For this review, take the finished solid that the model builds, in its own axes (mm). Give positions to 0.01 mm unless a question says otherwise; leave off trailing zeros. Order: outer loops, then holes, each group sorted by start corner. A loop starts at its lowest first (then second) coordinate and runs counter-clockwise, first axis right, second up. Notation, with made-up numbers: (82, 84.5) - (105, 84.5) arc R5 ccw to (105, 90.5) - close; hole circle Ø2 at (-20.75, -32.5). An arc over 180 degrees is marked (long way). Put each result on its own line as item: value. Start each with the question number.
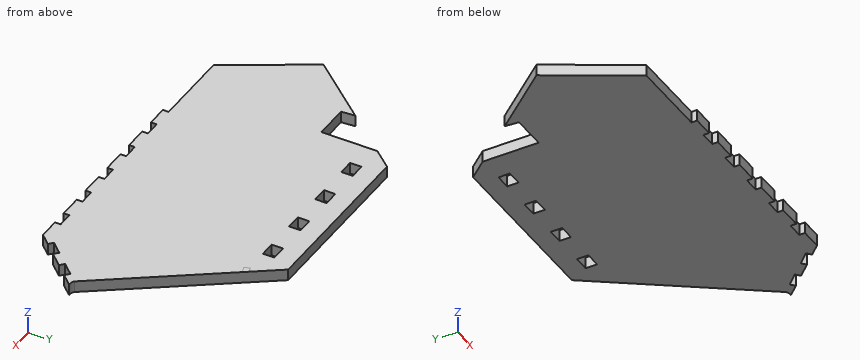
```python
from build123d import *

# Parameters (mm, degrees)
BOSS_EXTRU_1_DEPTH      = 6
ESQUISSE3_W             = 8
ESQUISSE3_H             = 3
ENL_V_MAT_EXTRU_1_DEPTH = 6
BOSS_EXTRU_2_DEPTH      = 6
ENL_V_MAT_EXTRU_2_DEPTH = 6
ENL_V_MAT_EXTRU_3_DEPTH = 10
ESQUISSE9_W             = 8
ESQUISSE9_H             = 6
ENL_V_MAT_EXTRU_4_DEPTH = 6
ENL_V_MAT_EXTRU_5_DEPTH = 10
ENL_V_MAT_EXTRU_6_DEPTH = 0.006


with BuildPart() as part:
    # Esquisse1 → Boss.-Extru.1 (new body)
    with BuildSketch(Plane.XY):
        Polygon((0, 0), (110, 0), (137.279934402, 29.254148065), (105.119046883, 134.447671221), (102.250132615, 133.570556107), (133.904617487, 30.033401375), (108.695562875, 3), (0, 3), align=None)
    extrude(amount=BOSS_EXTRU_1_DEPTH)

    # Esquisse3 → Enl_v. mat.-Extru.1 (cut)
    with BuildSketch(Plane(origin=(0, 0, 0), x_dir=(-1, 0, 0), z_dir=(0, 0, -1))):
        with Locations((-15, 1.5)):
            Rectangle(ESQUISSE3_W, ESQUISSE3_H)
        with Locations((-35, 1.5)):
            Rectangle(ESQUISSE3_W, ESQUISSE3_H)
        with Locations((-55, 1.5)):
            Rectangle(ESQUISSE3_W, ESQUISSE3_H)
        with Locations((-75, 1.5)):
            Rectangle(ESQUISSE3_W, ESQUISSE3_H)
        with Locations((-95, 1.5)):
            Rectangle(ESQUISSE3_W, ESQUISSE3_H)
        Polygon((-112.787553035, 7.38812221), (-114.98161414, 5.34212713), (-120.437601021, 11.192956742), (-118.243539916, 13.238951823), align=None)
        Polygon((-124.356640446, 19.794449553), (-126.550701551, 17.748454473), (-132.006688432, 23.599284086), (-129.812627327, 25.645279166), align=None)
        Polygon((-107.805195005, 115.400765743), (-110.674109273, 116.277880857), (-108.335135635, 123.928318905), (-105.466221367, 123.051203791), align=None)
        Polygon((-112.981575907, 96.082249217), (-115.850490175, 96.959364332), (-113.511516537, 104.609802379), (-110.642602269, 103.732687265), align=None)
        Polygon((-118.157956809, 76.763732692), (-121.026871077, 77.640847806), (-118.687897439, 85.291285854), (-115.818983171, 84.414170739), align=None)
        Polygon((-123.334337711, 57.445216166), (-126.203251979, 58.32233128), (-123.864278341, 65.972769328), (-120.995364073, 65.095654214), align=None)
        Polygon((-128.510718613, 38.12669964), (-131.379632881, 39.003814754), (-129.040659243, 46.654252802), (-126.171744975, 45.777137688), align=None)
    extrude(amount=-ENL_V_MAT_EXTRU_1_DEPTH, mode=Mode.SUBTRACT)


with BuildPart() as enl_v_mat_extru_1_piece_1:
    # of the separate pieces the step leaves, piece 1, a body of its own (enl_v_mat_extru_1_pieces)
    add(part.part.solids().sort_by_distance((132.006688432, 23.599284086, 0))[0])



with BuildPart() as enl_v_mat_extru_1_piece_2:
    # of the separate pieces the step leaves, piece 2, a body of its own (enl_v_mat_extru_1_pieces)
    add(part.part.solids().sort_by_distance((99, 0, 0))[0])


with BuildPart() as enl_v_mat_extru_1_piece_3:
    # of the separate pieces the step leaves, piece 3, a body of its own (enl_v_mat_extru_1_pieces)
    add(part.part.solids().sort_by_distance((39, 0, 0))[0])


with BuildPart() as enl_v_mat_extru_1_piece_4:
    # of the separate pieces the step leaves, piece 4, a body of its own (enl_v_mat_extru_1_pieces)
    add(part.part.solids().sort_by_distance((19, 0, 0))[0])


with BuildPart() as enl_v_mat_extru_1_piece_5:
    # of the separate pieces the step leaves, piece 5, a body of its own (enl_v_mat_extru_1_pieces)
    add(part.part.solids().sort_by_distance((59, 0, 0))[0])


with BuildPart() as enl_v_mat_extru_1_piece_6:
    # of the separate pieces the step leaves, piece 6, a body of its own (enl_v_mat_extru_1_pieces)
    add(part.part.solids().sort_by_distance((79, 0, 0))[0])


with BuildPart() as enl_v_mat_extru_1_piece_7:
    # of the separate pieces the step leaves, piece 7, a body of its own (enl_v_mat_extru_1_pieces)
    add(part.part.solids().sort_by_distance((0, 0, 0))[0])


with BuildPart() as enl_v_mat_extru_1_piece_8:
    # of the separate pieces the step leaves, piece 8, a body of its own (enl_v_mat_extru_1_pieces)
    add(part.part.solids().sort_by_distance((108.335135635, 123.928318905, 0))[0])


with BuildPart() as enl_v_mat_extru_1_piece_9:
    # of the separate pieces the step leaves, piece 9, a body of its own (enl_v_mat_extru_1_pieces)
    add(part.part.solids().sort_by_distance((120.437601021, 11.192956742, 0))[0])


with BuildPart() as enl_v_mat_extru_1_piece_1_1:
    add(enl_v_mat_extru_1_piece_1.part)

    add(enl_v_mat_extru_1_piece_2.part)  # Boss.-Extru.2 merges Enl_v. mat.-Extru.1 piece 2

    add(enl_v_mat_extru_1_piece_3.part)  # Boss.-Extru.2 merges Enl_v. mat.-Extru.1 piece 3

    add(enl_v_mat_extru_1_piece_4.part)  # Boss.-Extru.2 merges Enl_v. mat.-Extru.1 piece 4

    add(enl_v_mat_extru_1_piece_5.part)  # Boss.-Extru.2 merges Enl_v. mat.-Extru.1 piece 5

    add(enl_v_mat_extru_1_piece_6.part)  # Boss.-Extru.2 merges Enl_v. mat.-Extru.1 piece 6

    add(enl_v_mat_extru_1_piece_7.part)  # Boss.-Extru.2 merges Enl_v. mat.-Extru.1 piece 7

    add(enl_v_mat_extru_1_piece_9.part)  # Boss.-Extru.2 merges Enl_v. mat.-Extru.1 piece 9
    # Esquisse4 → Boss.-Extru.2 (add)
    with BuildSketch(Plane(origin=(0, 0, 0), x_dir=(-1, 0, 0), z_dir=(0, 0, -1))):
        Polygon((-39, 3), (0, 3), (41.304437125, 3), (66.304437125, 46.301270189), (-36.541580425, 168.868381088), (-133.904617487, 30.033401375), (-108.695562875, 3), (-51, 3), align=None)
    extrude(amount=-BOSS_EXTRU_2_DEPTH)


with BuildPart() as enl_v_mat_extru_2_tool:
    # Esquisse7 → Enl_v. mat.-Extru.2 (new body)
    with BuildSketch(Plane(origin=(0, 0, 0), x_dir=(-1, 0, 0), z_dir=(0, 0, -1))):
        with BuildLine():
            Line((-137.279934402, 29.254148065), (-105.119046883, 134.447671221))
            Line((-105.119046883, 134.447671221), (-102.250132615, 133.570556107))
            Line((-102.250132615, 133.570556107), (-133.904617487, 30.033401375))
            ThreePointArc((-133.904617487, 30.033401375), (-135.487875797, 29.191567999), (-137.279934402, 29.254148065))
        make_face()
    extrude(amount=-ENL_V_MAT_EXTRU_2_DEPTH)


with BuildPart() as enl_v_mat_extru_1_piece_1_2:
    add(enl_v_mat_extru_1_piece_1_1.part)

    # Enl_v. mat.-Extru.2: cut by enl_v_mat_extru_2_tool
    add(enl_v_mat_extru_2_tool.part, mode=Mode.SUBTRACT)

    # Esquisse8 → Enl_v. mat.-Extru.3 (cut)
    with BuildSketch(Plane(origin=(0, 0, 0), x_dir=(-1, 0, 0), z_dir=(0, 0, -1))):
        Polygon((12.854856434, 110), (-77.825155944, 110), (-36.541580425, 168.868381088), align=None)
    extrude(amount=-ENL_V_MAT_EXTRU_3_DEPTH, mode=Mode.SUBTRACT)

    # Esquisse9 → Enl_v. mat.-Extru.4 (cut)
    with BuildSketch(Plane.XY.offset(6)):
        with Locations((69, 97)):
            Rectangle(ESQUISSE9_W, ESQUISSE9_H)
        with Locations((45, 97)):
            Rectangle(ESQUISSE9_W, ESQUISSE9_H)
        with Locations((21, 97)):
            Rectangle(ESQUISSE9_W, ESQUISSE9_H)
        with Locations((-3, 97)):
            Rectangle(ESQUISSE9_W, ESQUISSE9_H)
    extrude(amount=-ENL_V_MAT_EXTRU_4_DEPTH, mode=Mode.SUBTRACT)

    # Esquisse10 → Enl_v. mat.-Extru.5 (cut)
    with BuildSketch(Plane.XY.offset(6)):
        Polygon((-21, 71), (-21, 100.292995893), (-39.57964678, 78.150635095), (-39, 71), align=None)
    extrude(amount=-ENL_V_MAT_EXTRU_5_DEPTH, mode=Mode.SUBTRACT)

    # Esquisse11 → Enl_v. mat.-Extru.6 (cut)
    with BuildSketch(Plane.XY.offset(6)):
        Polygon((86.271198829, 91.64198356), (89.917576683, 92.756793146), (88.105999998, 95.340013841), (85.394083714, 94.510897828), align=None)
    extrude(amount=-ENL_V_MAT_EXTRU_6_DEPTH, mode=Mode.SUBTRACT)


with BuildPart() as enl_v_mat_extru_1_piece_8_1:
    add(enl_v_mat_extru_1_piece_8.part)

    # Enl_v. mat.-Extru.2: cut by enl_v_mat_extru_2_tool
    add(enl_v_mat_extru_2_tool.part, mode=Mode.SUBTRACT)


solid = enl_v_mat_extru_1_piece_1_2.part
```
1. Add section A-A, the plane z = 2.8. Count the separate pieces of the cut face and the enclosed holes in it, then the cut area to 3 significant figures.
2. Add section C-C, the plane y = 83. Give the boundary of the cut face in (x, z), then the cut area to 3 significant figures.
3. Add section B-B, the plane x = -32.5. Give the boundary of the cut face in (y, z), then the cut area to 3 significant figures.
4. Clearance check with flat-ended pins moving along their axes: pin 1 (1.8 mm diameter, centred on x = 15.5, z = 3, fed in from -Y); pin 2 (2.5 mm diameter, centred on y = 1.5, z = 2.5, fed in from -X); pin 3 (3.5 mm diameter, centred on y = 1, z = 2.5, fed in from +X). State where each tip first meets the part, or that it passes through.
5. Wall thickness on line 1 (Y direction, x = 22.5, z = 3.95); line 2 (Y direction, x = 57.5, z = 5.55); line 3 (X direction, y = 73, z = 2.9): over which ranges is each line inside the solid? List them lowest first. Write a range as from..to.
Found:
1. separate pieces: 1
1. enclosed holes: 4
1. area: 16,300 mm^2
2. outline: (-21, 0) - (96.76, 0) - (96.76, 6) - (-21, 6) - close
2. area: 707 mm^2
3. outline: (3, 0) - (71, 0) - (71, 6) - (3, 6) - close
3. area: 408 mm^2
4. pin 1: stops at y = 3
4. pin 2: stops at x = 0
4. pin 3: stops at x = 112.56
5. line 1: y = 0..94, 100..110
5. line 2: y = 3..110
5. line 3: x = -43.9..-39.16, -21..103.77
